Autodesk Inventor part; units mm, degrees
ref_plane "Start plane" through (0, 0, -10.521) normal (0, 0, 1) x (1, 0, 0)
ref_plane "End plane" through (0, 0, 584.2) normal (0, 0, 1) x (1, 0, 0)
ref_plane "Work Plane3" through (50.8, 38.1, -10.521) normal (-0.3827, 0, -0.9239) x (-0.9239, 0, 0.3827)
ref_plane "Start plane" through (0, 0, -10.521) normal (0, 0, 1) x (1, 0, 0)
ref_plane "End plane" through (0, 0, 584.2) normal (0, 0, 1) x (1, 0, 0)
sketch "Sketch" plane through (0, 0, 0) normal (0, 0, 1) x (1, 0, 0)
  line L0 (0, 76.2) -> (0, 0)
  line L1 (0, 0) -> (50.8, 0)
  line L2 (50.8, 0) -> (50.8, 2.7625)
  line L3 (48.8, 4.7625) -> (12.6365, 4.7625)
  line L4 (4.7625, 12.6365) -> (4.7625, 74.2)
  line L5 (2.7625, 76.2) -> (0, 76.2)
  line L6 (-7.0414, 0) -> (21.5385, 0) construction
  line L7 (0, -8.0414) -> (0, 34.5385) construction
  arc A0 (4.7625, 12.6365) -> (12.6365, 4.7625) centre (12.6365, 12.6365) ccw
  arc A1 (50.8, 2.7625) -> (48.8, 4.7625) centre (48.8, 2.7625) ccw
  arc A2 (4.7625, 74.2) -> (2.7625, 76.2) centre (2.7625, 74.2) ccw
  line L8 (0, 93.5453) -> (0, -24.9725) construction
  line L9 (-18.6925, 0) -> (62.8653, 0) construction
  point P0 (50.8, 4.7625)
  point P1 (4.7625, 4.7625)
  point P2 (4.7625, 76.2)
  dimension "d12" = 4.7625
  dimension "d13" = 76.2
  dimension "d14" = 50.8
  dimension "d15" = 0
  dimension "d16" = 4.7625
  dimension "d17" = 0
  dimension "d18" = 7.874
  dimension "d19" = 2
extrude "Body" add sketch "Sketch" along normal up to surface (594.721 mm away) from surface at -10.521
sketch "Sketch3" plane through (0, 0, 0) normal (0, 0, 1) x (1, 0, 0)
  line L0 (0, 0) -> (10, 0)
ref_plane "Work Plane5" through (0, 0, 0) normal (0, -1, 0) x (1, 0, 0)
sketch "Sketch4" plane through (0, 0, 0) normal (0, -1, 0) x (1, 0, 0)
  line L0 (-2, -10.521) -> (12, -10.521)
  line L1 (-2, 584.2) -> (12, 584.2)
  dimension "d23" = 594.721
ref_plane "Work Plane3" through (50.8, 38.1, -10.521) normal (-0.3827, 0, -0.9239) x (-0.9239, 0, 0.3827)
split "Split1" plane through (50.8, 38.1, -10.521) removes the side toward (-0.3827, 0, -0.9239)
ref_plane "Work Plane4" through (130.175, 0, 584.2) normal (0, 0, 1) x (1, 0, 0)
split "Split2" plane through (130.175, 0, 584.2) removes the side toward (0, 0, 1)
equation "\"d12\" = G_T"
equation "\"d13\" = G_H"
equation "\"d14\" = G_W"
equation "\"d16\" = G_T"
equation "\"d18\" = G_IR"
equation "\"d4\" = G_L"
equation "\"G_W\" = 50.8"
equation "\"G_H\" = 76.2"
equation "\"G_T\" = 4.7625"
equation "\"G_ER\" = 4.064"
equation "\"G_IR\" = 7.874"
equation "\"G_L\" = d23"
equation "\"ex\" = 0"
equation "\"ey\" = 0"
equation "\"G_OFFSET_START\" = 10.52102"
equation "\"G_OFFSET_END\" = -25.4"
equation "\"d20\" = -G_OFFSET_START"
equation "\"d21\" = G_OFFSET_END + B_L"
equation "\"B_L\" = 609.6"
properties part number "ANSI L 3 x 2 x 3_16 00000003"
The model under review builds one solid part; all positions refer to its coordinate system, in mm. A direction names the side the tool comes from. Round coordinates to 2 decimals unless told otherwise and drop trailing zeros. Order: outer loops, then holes, each group sorted by start corner. A loop starts at its lowest first (then second) coordinate and runs counter-clockwise, first axis right, second up.
(1) Wall thickness on L1, parallel to X at y = 54, z = 19.5; L2, parallel to Z at x = 3, y = 23: over which ranges is each line inside the solid? List them lowest first.
Working result:
L1: x = 0 to 4.76
L2: z = 9.28 to 584.2
(2) Take a section at B-B, the plane y = 40.5. State the section outline as (x, z) points, plus the area to 3 significant figures.
Working result:
outline: (0, 10.52) - (4.76, 8.55) - (4.76, 584.2) - (0, 584.2) - close
area: 2,740 mm2
(3) Take a section at A-A, the plane z = 235. State the section outline as (x, y) points, plus the area to 3 significant figures.
Working result:
outline: (0, 0) - (50.8, 0) - (50.8, 2.76) arc R2 ccw to (48.8, 4.76) - (12.64, 4.76) arc R7.87 cw to (4.76, 12.64) - (4.76, 74.2) arc R2 ccw to (2.76, 76.2) - (0, 76.2) - close
area: 594 mm2
(4) Take a section at C-C, the plane x = 24.5. State the section outline as (y, z) points, plus the area to 3 significant figures.
Working result:
outline: (0, 0.37) - (4.76, 0.37) - (4.76, 584.2) - (0, 584.2) - close
area: 2,780 mm2
(5) For P1, Ø3, axis at y = 11.5, z = 125, coming from the +X side; P2, Ø11, axis at x = 39.5, z = 415, coming from the +Y side; P3, Ø1.5, axis at x = 6.5, z = 402.5, coming from the +Y side, all flat-tipped, find the tip position at first contact; note any pin that passes through.
Working result:
P1: stops at x = 5.22
P2: stops at y = 4.76
P3: stops at y = 8.82
(6) Tool access review of faces 1 (the face through (4.59, 21.34, 8.62)), 2 (the face through (31, 4.762, 283)): name each direction out of +Z, -Z, +X, -X, +Y, -Y from which nothing blocks a thin tool from reaching the whole face with its end or side.
Working result:
face 1: -Z, -X, +Y, -Y
face 2: +Z, -Z, +X, +Y
